Source: CAD feature listing. Evaluate the final solid. Frame: model axes, mm. A direction names the side the tool comes from. Coordinates: 2 decimals unless noted, no trailing zeros. Loops run counter-clockwise (first coordinate to the right, second up) from the corner with the lowest first, then second, coordinate; pieces in that order, holes last.
Item 1: Section query B-B, the plane y = 0. Return the cut outline in (x, z).
Item 2: Pin query (flat end, axial travel): pin 1 Ø11.5 at (x, y) = (26.5, 0) entering from -Z; pin 2 Ø8 at (x, y) = (-26.81, 22.5) entering from +Z; pin 3 Ø1 at (x, z) = (9.5, 1) entering from +Y; pin 4 Ø1 at (x, z) = (14, 1.5) entering from -Y. Return the tip coordinate at first contact, or that it passes through.
Item 3: Line query: probe 1 along X at (y, z) = (-3, 0.8); probe 2 along X at (y, z) = (-0.5, 0.25); probe 3 along Y at (x, z) = (-31, 0.55). Output: solid intervals per line, ascending.
Item 4: Section query C-C, the plane z = 1.5. Return the cut outline in (x, y).
Item 5: Reachability of faces 1 (the flat face through (13, -6, 1)), 2 (the cylindrical face through (-7.45, -1.73, 1.01)), 3 (the cylindrical face through (2.584, 7.041, 0.986)) from +Z, -Z, +X, -X, +Y, -Y: full face, straight path, thin tool, end or side. Return the list, or none.
Item 6: Section query A-A, the plane x = 26.5. Return the cut outline in (y, z), then the cut area to 3 significant figures.
Item 7: Pull-direction query (Y, two-part tool) for faces 4 (the cylindrical face through (-22.285, 20.621, 0.986)), 5 (the cylindrical face through (21.883, -6.106, 1.014)), 6 (the cylindrical face through (-32.4, 27.5, 1)), 7 (the cylindrical face through (21.605, 0.215, 0.986)); classes: +Y half, -Y half, draft (parallel to the pull), parting line (faces both ways), or undercut.
Item 8: Section query D-D, the plane x = 2. Return the cut outline in (y, z), then the cut area to 3 significant figures.
```python
from build123d import *

# Parameters (mm, degrees)
SKETCH1_R           = 4.9
BOSS_EXTRUDE1_DEPTH = 2
FILLET1_R           = 3


with BuildPart() as part:
    # Sketch1 → Boss-Extrude1 (new body)
    with BuildSketch(Plane.XY):
        with BuildLine():
            Line((4.5, -6), (22, -6))
            ThreePointArc((22, -6), (34, 0), (22, 6))
            Line((22, 6), (4.5, 6))
            ThreePointArc((4.5, 6), (2.565151075, 7.047694656), (0.409525664, 7.488810902))
            Line((0.409525664, 7.488810902), (-19.507629857, 24.201288754))
            ThreePointArc((-19.507629857, 24.201288754), (-32.556888833, 27.318473412), (-27.221081173, 15.008755437))
            Line((-27.221081173, 15.008755437), (-7.303925652, -1.703722415))
            ThreePointArc((-7.303925652, -1.703722415), (-2.565151075, -7.047694656), (4.5, -6))
        make_face()
        Circle(SKETCH1_R, mode=Mode.SUBTRACT)
        with Locations((26.5, 0)):
            Circle(SKETCH1_R, mode=Mode.SUBTRACT)
        with Locations((-26.811555509, 22.497566339)):
            Circle(SKETCH1_R, mode=Mode.SUBTRACT)
    extrude(amount=BOSS_EXTRUDE1_DEPTH)

    # Fillet1
    fillet1_edges = [part.edges().sort_by_distance(p)[0] for p in [
        (-19.507629857, 24.201288754, 1),
        (0.409525664, 7.488810902, 1),
        (4.5, 6, 1),
        (22, 6, 1),
        (22, -6, 1),
        (4.5, -6, 1),
        (-7.303925652, -1.703722415, 1),
        (-27.221081173, 15.008755437, 1),
    ]]
    fillet(fillet1_edges, radius=FILLET1_R)


solid = part.part
```
Verdict:
1. outline: (-9.33, 0) - (-4.9, 0) - (-4.9, 2) - (-9.33, 2) - close; (4.9, 0) - (21.6, 0) - (21.6, 2) - (4.9, 2) - close; (31.4, 0) - (34, 0) - (34, 2) - (31.4, 2) - close
2. pin 1: stops at z = 0
2. pin 2: passes through
2. pin 3: stops at y = 6
2. pin 4: stops at y = -6
3. probe 1: x = -6.87 to -3.87, 3.87 to 22.63, 30.37 to 33.37
3. probe 2: x = -8.74 to -4.87, 4.87 to 21.63, 31.37 to 33.98
3. probe 3: y = 16.28 to 19.95, 25.04 to 28.72
4. outline: (-27.98, 15.09) arc R3 cw to (-26.53, 14.42) - (-8, -1.12) arc R3 cw to (-7.09, -2.44) arc R7.5 ccw to (3.86, -6.43) arc R3 cw to (5.41, -6) - (21.09, -6) arc R3 cw to (22.64, -6.43) arc R7.5 ccw (long way) to (22.64, 6.43) arc R3 cw to (21.09, 6) - (5.41, 6) arc R3 cw to (3.86, 6.43) arc R7.5 ccw to (1.17, 7.41) arc R3 cw to (-0.29, 8.07) - (-18.81, 23.62) arc R3 cw to (-19.72, 24.94) arc R7.5 ccw (long way) to start; hole circle Ø9.8 at (-26.81, 22.5); hole circle Ø9.8 at (0, 0); hole circle Ø9.8 at (26.5, 0)
5. face 1: +Z, -Z, -Y
5. face 2: +Z, -Z, -X, -Y
5. face 3: +Z, -Z, +Y
6. outline: (-7.5, 0) - (-4.9, 0) - (-4.9, 2) - (-7.5, 2) - close; (4.9, 0) - (7.5, 0) - (7.5, 2) - (4.9, 2) - close
6. area: 10.4 mm2
7. face 4: undercut
7. face 5: -Y half
7. face 6: parting line
7. face 7: undercut
8. outline: (-7.23, 0) - (-4.47, 0) - (-4.47, 2) - (-7.23, 2) - close; (4.47, 0) - (7.23, 0) - (7.23, 2) - (4.47, 2) - close
8. area: 11.0 mm2
